For this review, take the finished solid that the model builds, in its own axes (mm). Face numbers are marked on the shaded views. Give positions to 0.01 mm unless a question says otherwise; leave off trailing zeros. Order: outer loops, then holes, each group sorted by start corner. A loop starts at its lowest first (then second) coordinate and runs counter-clockwise, first axis right, second up. Notation, with made-up numbers: (86, 44.5) - (133, 44.5) arc R21 ccw to (133, 68.5) - close; hole circle Ø11 at (9, 43). An arc over 180 degrees is marked (long way). Use a Markdown table: item, result. Add a question column.
1) Clearance check with a flat-ended pin moving along its axis: P1, Ø2.5, axis at x = 0, z = 0, coming from the +Y side. State where the tip first meets the part, or that it passes through.
2) Wall thickness on L1, parallel to Z at x = 0, y = 1.4; L2, parallel to X at y = 0.2, z = -0.1; L3, parallel to Z at x = 14.25, y = 0.2: over which ranges is each line inside the solid? List them lowest first.
3) Mouldability with a two-part tool opening along X and no side actions: class the marked faces 1, 2, 3 and 4 as released by +X, released by -X, zero draft, split by the parting line, or undercut.
4) We need section A-A on x = 14.8. Write out the cut boundary in (y, z).
5) We need section B-B on z = 0. Write out the cut boundary in (x, y), then the cut area to 3 significant figures.
6) We need section C-C on y = 0.5. Write out the cut boundary in (x, z), then the cut area to 3 significant figures.
Autodesk Inventor part; units mm, degrees
ref_plane "YZ Plane" through (0, 0, 0) normal (1, 0, 0) x (0, 1, 0)
ref_plane "XZ Plane" through (0, 0, 0) normal (0, 1, 0) x (-1, 0, 0)
ref_plane "XY Plane" through (0, 0, 0) normal (0, 0, 1) x (1, 0, 0)
sketch "スケッチ1" plane through (0, 0, 0) normal (0, 1, 0) x (-1, 0, 0)
  line L0 (0, 0) -> (-14.8, 0)
  circle A0 centre (-14.8, 0) radius 1.5
  circle A1 centre (0, 0) radius 1.5
  line L1 (-18.4, 3) -> (3.6, 3)
  line L2 (3.6, 3) -> (3.6, -3)
  line L3 (3.6, -3) -> (-18.4, -3)
  line L4 (-18.4, -3) -> (-18.4, 3)
  line L5 (-18.4, 3) -> (3.6, -3) construction
  line L6 (3.6, 3) -> (-18.4, -3) construction
  point P0 (-7.4, 0)
  dimension "d0" = 14.8
  dimension "d1" = 3
  dimension "d2" = 3
  dimension "d3" = 22
  dimension "d4" = 6
extrude "押し出し1" add sketch "スケッチ1" along normal blind 3
properties part number "知能ロボコン砲身止め" material "ABS プラスチック"
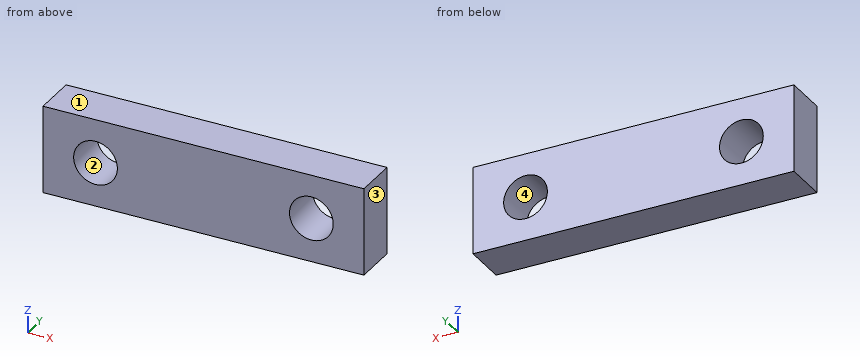
Checked values:
| question | item | result |
|---|---|---|
| 1 | P1 | through |
| 2 | L1 | -3 to -1.5, 1.5 to 3 |
| 2 | L2 | -3.6 to -1.5, 1.5 to 13.3, 16.3 to 18.4 |
| 2 | L3 | -3 to -1.4, 1.4 to 3 |
| 3 | face 1 | zero draft |
| 3 | face 2 | undercut |
| 3 | face 3 | released by +X |
| 3 | face 4 | undercut |
| 4 | outline | (0, -3) - (3, -3) - (3, -1.5) - (0, -1.5) - close; (0, 1.5) - (3, 1.5) - (3, 3) - (0, 3) - close |
| 5 | outline | (-3.6, 0) - (-1.5, 0) - (-1.5, 3) - (-3.6, 3) - close; (1.5, 0) - (13.3, 0) - (13.3, 3) - (1.5, 3) - close; (16.3, 0) - (18.4, 0) - (18.4, 3) - (16.3, 3) - close |
| 5 | area | 48.0 mm² |
| 6 | outline | (-3.6, -3) - (18.4, -3) - (18.4, 3) - (-3.6, 3) - close; hole circle Ø3 at (0, 0); hole circle Ø3 at (14.8, 0) |
| 6 | area | 118 mm² |
